The listing builds one solid part. Answer for the finished solid, in the listing's coordinates (mm). Face numbers are marked on the shaded views. A direction names the side the tool comes from. Give positions to 0.01 mm unless a question says otherwise; leave off trailing zeros. Write each loop counter-clockwise with the first axis right and the second up, starting at its lowest first coordinate (ties: lowest second). Pieces come first, ordered by that corner, then holes. Notation, with made-up numbers: (-37.75, -30) - (-30.75, -30) arc R31 ccw to (-30.75, -4) - close; hole circle Ø1 at (-9.5, 12.25). An arc over 180 degrees is marked (long way). Return JSON: item names as keys, results as strings.
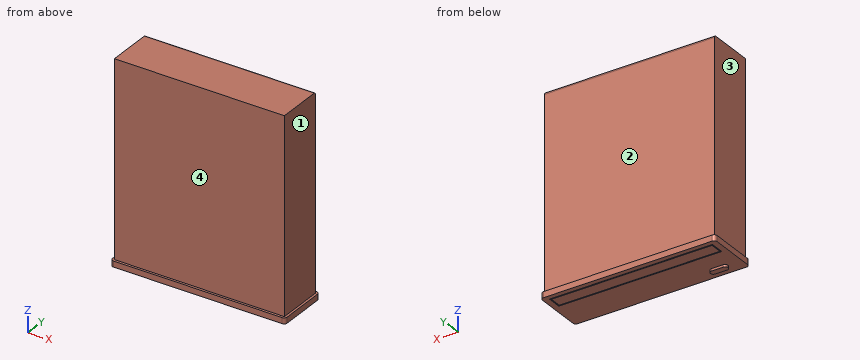
from build123d import *

# Parameters (mm, degrees)
F0_W     = 145
F0_H     = 40
F1_DEPTH = 165
F2_R     = 2
F4_DEPTH = 5
F6_DEPTH = 0.2
F7_DEPTH = 1
F9_DEPTH = 2


with BuildPart() as f1:
    # F0 (on Top) → F1 (new body)
    with BuildSketch(Plane.XY):
        with Locations((21.1617818475, 12.8752994537)):
            Rectangle(F0_W, F0_H)
    extrude(amount=F1_DEPTH)

    # F2
    f2_edges = [f1.edges().sort_by_distance(p)[0] for p in [
        (21.161782, 32.875299, 165),
    ]]
    fillet(f2_edges, radius=F2_R)

    # F3 (on face) → F4 (join)
    with BuildSketch(Plane(origin=(0, 0, 0), x_dir=(1, 0, 0), z_dir=(0, 0, -1))):
        with BuildLine():
            Line((-53.3382181525, 6.6247005463), (-53.3382181525, -12.8752994537))
            Line((-53.3382181525, -12.8752994537), (-53.3382181525, -32.3752994537))
            ThreePointArc((-53.3382181525, -32.3752994537), (-52.6059851055, -34.1430664067), (-50.8382181525, -34.8752994537))
            Line((-50.8382181525, -34.8752994537), (45.6353314221, -34.8752994537))
            Line((45.6353314221, -34.8752994537), (93.1617818475, -34.8752994537))
            ThreePointArc((93.1617818475, -34.8752994537), (94.9295488004, -34.1430664067), (95.6617818475, -32.3752994537))
            Line((95.6617818475, -32.3752994537), (95.6617818475, -12.8752994537))
            Line((95.6617818475, -12.8752994537), (95.6617818475, 6.6247005463))
            ThreePointArc((95.6617818475, 6.6247005463), (94.9295488004, 8.3924674992), (93.1617818475, 9.1247005463))
            Line((93.1617818475, 9.1247005463), (22.451678291, 9.1247005463))
            Line((22.451678291, 9.1247005463), (-50.8382181525, 9.1247005463))
            ThreePointArc((-50.8382181525, 9.1247005463), (-52.6059851055, 8.3924674992), (-53.3382181525, 6.6247005463))
        make_face()
    extrude(amount=F4_DEPTH)

    # F5 (on face) → F6 (join)
    with BuildSketch(Plane(origin=(0, 0, -5), x_dir=(1, 0, 0), z_dir=(0, 0, -1))):
        Polygon((-48.3382181525, -30.8752994537), (29.9128331244, -30.8752994537), (41.8360643089, -30.8752994537), (41.8360643089, -29.8752994537), (-47.3382181525, -29.8752994537), (-47.3382181525, -24.8752994537), (-48.3382181525, -24.8752994537), align=None)
        Polygon((41.8360643089, -29.8752994537), (41.8360643089, -30.8752994537), (90.6617818475, -30.8752994537), (90.6617818475, -27.4621471763), (90.6617818475, -24.8752994537), (89.6617818475, -24.8752994537), (89.6617818475, -29.8752994537), align=None)
        Polygon((-48.3382181525, -20.8752994537), (-48.3382181525, -24.8752994537), (-47.3382181525, -24.8752994537), (-47.3382181525, -19.8752994537), (26.0328520089, -19.8752994537), (26.0328520089, -18.8752994537), (-48.3382181525, -18.8752994537), align=None)
        Polygon((89.6617818475, -24.8752994537), (90.6617818475, -24.8752994537), (90.6617818475, -18.8752994537), (26.0328520089, -18.8752994537), (26.0328520089, -19.8752994537), (89.6617818475, -19.8752994537), align=None)
    extrude(amount=F6_DEPTH)

    # F7 (cut): a face of the model
    f7_faces = [f1.faces().sort_by_distance(p)[0] for p in [
        (21.1617818475, 30.7357824297, -5.2),
    ]]
    extrude(f7_faces, amount=-F7_DEPTH, mode=Mode.SUBTRACT)

    # F8 (on face) → F9 (join)
    with BuildSketch(Plane(origin=(0, 0, -5), x_dir=(1, 0, 0), z_dir=(0, 0, -1))):
        with BuildLine():
            ThreePointArc((-41.3382181525, -0.3752994537), (-40.6059851055, -2.1430664067), (-38.8382181525, -2.8752994537))
            Line((-38.8382181525, -2.8752994537), (-28.8382181525, -2.8752994537))
            ThreePointArc((-28.8382181525, -2.8752994537), (-27.0704511996, -2.1430664067), (-26.3382181525, -0.3752994537))
            ThreePointArc((-26.3382181525, -0.3752994537), (-27.0704511996, 1.3924674992), (-28.8382181525, 2.1247005463))
            Line((-28.8382181525, 2.1247005463), (-38.8382181525, 2.1247005463))
            ThreePointArc((-38.8382181525, 2.1247005463), (-40.6059851055, 1.3924674992), (-41.3382181525, -0.3752994537))
        make_face()
    extrude(amount=F9_DEPTH)


solid = f1.part
Item 1: A cutting plane is placed at B-B on x = -34.5. Determine the outline of the cut face in (y, z).
Answer below:
{"outline": "(-9.12, -5) - (-2.12, -5) - (-2.12, -7) - (2.88, -7) - (2.88, -5) - (18.88, -5) - (18.88, -4.2) - (19.88, -4.2) - (19.88, -5) - (29.88, -5) - (29.88, -4.2) - (30.88, -4.2) - (30.88, -5) - (34.88, -5) - (34.88, 0) - (32.88, 0) - (32.88, 163) arc R2 ccw to (30.88, 165) - (-7.12, 165) - (-7.12, 0) - (-9.12, 0) - close"}
Item 2: For the marked faces 1, 2, 3 and 4, determine the directions among +Z, -Z, +X, -X, +Y, -Y from which every point of the face is accessible in a straight line to the end or side of a thin tool.
Answer below:
{"face 1": "+Z, +X, +Y, -Y", "face 2": "+Z, +X, -X, +Y", "face 3": "+Z, -X, +Y, -Y", "face 4": "+Z, +X, -X, -Y"}
Item 3: A cutting plane is placed at D-D on z = 77. Determine the outline of the cut face in (x, y), then the cut area to 3 significant figures.
Answer below:
{"outline": "(-51.34, -7.12) - (93.66, -7.12) - (93.66, 32.88) - (-51.34, 32.88) - close", "area": "5,800 mm²"}
Item 4: A cutting plane is placed at A-A on y = 5.5. Determine the outline of the cut face in (x, z).
Answer below:
{"outline": "(-53.34, -5) - (95.66, -5) - (95.66, 0) - (93.66, 0) - (93.66, 165) - (-51.34, 165) - (-51.34, 0) - (-53.34, 0) - close"}
Item 5: A cutting plane is placed at C-C on y = 25.5. Determine the outline of the cut face in (x, z), then the cut area to 3 significant figures.
Answer below:
{"outline": "(-53.34, -5) - (-48.34, -5) - (-48.34, -4.2) - (-47.34, -4.2) - (-47.34, -5) - (89.66, -5) - (89.66, -4.2) - (90.66, -4.2) - (90.66, -5) - (95.66, -5) - (95.66, 0) - (93.66, 0) - (93.66, 165) - (-51.34, 165) - (-51.34, 0) - (-53.34, 0) - close", "area": "24,700 mm²"}
Item 6: Flat-ended cylindrical pins translate along their axes: P1, Ø8, axis at y = 6, z = 76, coming from the -X side; P2, Ø2, axis at y = 24.5, z = 139, coming from the +X side; P3, Ø8, axis at x = 22, z = 57, coming from the -Y side. Find the tip coordinate at first contact, or state that the pin passes through.
Answer below:
{"P1": "stops at x = -51.34", "P2": "stops at x = 93.66", "P3": "stops at y = -7.12"}
Item 7: Consider L1, parallel to Z at x = 44.5, y = 29; L2, parallel to Z at x = -2.5, y = 19.5; L3, parallel to X at y = 13, z = 126.5. Determine where each line is inside the solid, lowest interval first.
Answer below:
{"L1": "z = -5 to 165", "L2": "z = -4.2 to 165", "L3": "x = -51.34 to 93.66"}
